from build123d import *

# Parameters (mm, degrees)
CROQUIS1_R              = 2
SALIENTE_EXTRUIR1_DEPTH = 10
REDONDEO2_R             = 10


with BuildPart() as part:
    # Croquis1 → Saliente-Extruir1 (new body)
    with BuildSketch(Plane.XY):
        with BuildLine():
            Line((12.815, 7.35), (49.185, 7.35))
            Line((49.185, 7.35), (62, 4))
            ThreePointArc((62, 4), (66, 0), (62, -4))
            Line((62, -4), (49.185, -7.35))
            Line((49.185, -7.35), (12.815, -7.35))
            Line((12.815, -7.35), (0, -4))
            ThreePointArc((0, -4), (-4, 0), (0, 4))
            Line((0, 4), (12.815, 7.35))
        make_face()
        Circle(CROQUIS1_R, mode=Mode.SUBTRACT)
        with Locations((62, 0)):
            Circle(CROQUIS1_R, mode=Mode.SUBTRACT)
    extrude(amount=SALIENTE_EXTRUIR1_DEPTH)

    # Redondeo2
    redondeo2_edges = [part.edges().sort_by_distance(p)[0] for p in [
        (12.815, 7.35, 5),
        (49.185, 7.35, 5),
        (49.185, -7.35, 5),
        (12.815, -7.35, 5),
    ]]
    fillet(redondeo2_edges, radius=REDONDEO2_R)


solid = part.part
Read the model definition and answer for the solid it produces. Units are mm, in the model's axes. Coordinates: 2 decimals unless noted, no trailing zeros. Order: outer loops, then holes, each group sorted by start corner. A loop starts at its lowest first (then second) coordinate and runs counter-clockwise, first axis right, second up. Notation, with made-up numbers: (34.5, 66.25) - (49.5, 66.25) arc R23 cw to (49.5, 94.25) - close; hole circle Ø10 at (47.5, -15). An arc over 180 degrees is marked (long way). Use one line per item in the form item = value.
(1) Section B-B, the plane z = 1 is taken. Give the vertices of the cut face in (x, y), then the cut area to 3 significant figures.
Computed values:
outline = (0, -4) - (11.57, -7.02) arc R10 ccw to (14.1, -7.35) - (47.9, -7.35) arc R10 ccw to (50.43, -7.02) - (62, -4) arc R4 ccw to (62, 4) - (50.43, 7.02) arc R10 ccw to (47.9, 7.35) - (14.1, 7.35) arc R10 ccw to (11.57, 7.02) - (0, 4) arc R4 ccw to start; hole circle Ø4 at (0, 0); hole circle Ø4 at (62, 0)
area = 850 mm²
(2) Section A-A, the plane y = 0 is taken. Give the vertices of the cut face in (x, z).
Computed values:
outline = (-4, 0) - (-2, 0) - (-2, 10) - (-4, 10) - close; (2, 0) - (60, 0) - (60, 10) - (2, 10) - close; (64, 0) - (66, 0) - (66, 10) - (64, 10) - close
(3) For a pull along X with two mould halves and no side action, classify faces 1 (the face through (31, 0, 0)), 2 (the face through (49.16, 7.27, 5.07)), 3 (the face through (60, 0, 5)) as pulls with the +X half, pulls with the -X half, needs draft (parallel to the pull), parting line crosses it, or undercut.
Computed values:
face_1 = needs draft
face_2 = pulls with the +X half
face_3 = undercut
(4) Straight lines are drawn through the part: L1, parallel to Y at x = 0, z = 5; L2, parallel to X at y = 1.5, z = 8; L3, parallel to Y at x = 14, z = 8.5. For each, find the intervals that lie inside material, in ascending order.
Computed values:
L1 = -4 to -2, 2 to 4
L2 = -3.71 to -1.32, 1.32 to 60.68, 63.32 to 65.71
L3 = -7.35 to 7.35
(5) Section D-D, the plane y = 3 is taken. Give the vertices of the cut face in (x, z).
Computed values:
outline = (-2.65, 0) - (64.65, 0) - (64.65, 10) - (-2.65, 10) - close
(6) Given pin 1 Ø2.5 at (x, y) = (0, 0) entering from -Z; pin 2 Ø1.5 at (y, z) = (3, 8.5) entering from -X; pin 3 Ø4 at (y, z) = (-5, 3) entering from +X; pin 4 Ø1 at (x, z) = (56.5, 7.5) entering from -Y, each flat-ended and moving along its own axis, determine where each tip first touches the part or whether it passes through.
Computed values:
pin_1 = through
pin_2 = -3.31
pin_3 = 64.65
pin_4 = -5.57
(7) Section C-C, the plane x = 57 is taken. Give the vertices of the cut face in (y, z).
Computed values:
outline = (-5.31, 0) - (5.31, 0) - (5.31, 10) - (-5.31, 10) - close
